```python
from build123d import *

# Parameters (mm, degrees)
F1_DEPTH = 12.7
F2_SIZE  = 12.7
F4_R     = 1.9812
F4_R_2   = 2.067369
F4_R_3   = 1.772036
F4_R_4   = 2.051504
F5_DEPTH = 12.701
F6_R     = 2.54
F7_DEPTH = 12.701


with BuildPart() as f1:
    # F0 (on Front) → F1 (new body)
    with BuildSketch(Plane.XZ):
        with BuildLine():
            Line((0, 25.4), (0, 0))
            Line((0, 0), (762, 0))
            Line((762, 0), (762, 562.7624))
            Line((762, 562.7624), (0, 562.7624))
            Line((0, 562.7624), (0, 537.3624))
            ThreePointArc((0, 537.3624), (-37.197439, 447.559839), (-127, 410.3624))
            Line((-127, 410.3624), (-711.2, 410.3624))
            Line((-711.2, 410.3624), (-711.2, 152.4))
            Line((-711.2, 152.4), (-127, 152.4))
            ThreePointArc((-127, 152.4), (-37.197439, 115.202561), (0, 25.4))
        make_face()
    extrude(amount=F1_DEPTH)

    # F2
    f2_edges = [f1.edges().sort_by_distance(p)[0] for p in [
        (-711.2, -6.35, 410.3624),
        (-711.2, -6.35, 152.4),
        (0, -6.35, 0),
        (0, -6.35, 562.7624),
        (762, -6.35, 562.7624),
        (762, -6.35, 0),
    ]]
    chamfer(f2_edges, length=F2_SIZE)

    # F4 (on face) → F5 (cut, through all)
    with BuildSketch(Plane.XZ.offset(12.7)):
        with Locations((713.74, 7.62)):
            Circle(F4_R)
        with Locations((739.14, 7.62)):
            Circle(F4_R_2)
        with Locations((739.14, 50.8)):
            Circle(F4_R_3)
        with Locations((713.74, 50.8)):
            Circle(F4_R_4)
        with Locations((713.74, 555.1424)):
            Circle(F4_R)
        with Locations((739.14, 555.1424)):
            Circle(F4_R)
        with Locations((739.14, 511.9624)):
            Circle(F4_R)
        with Locations((713.74, 511.9624)):
            Circle(F4_R)
        with Locations((22.86, 555.1424)):
            Circle(F4_R)
        with Locations((48.26, 555.1424)):
            Circle(F4_R)
        with Locations((48.26, 511.9624)):
            Circle(F4_R)
        with Locations((22.86, 511.9624)):
            Circle(F4_R)
        with Locations((22.86, 7.62)):
            Circle(F4_R)
        with Locations((48.26, 7.62)):
            Circle(F4_R)
        with Locations((48.26, 48.8188)):
            Circle(F4_R)
        with Locations((22.86, 48.8188)):
            Circle(F4_R)
    extrude(amount=-F5_DEPTH, mode=Mode.SUBTRACT)

    # F6 (on face) → F7 (cut, through all)
    with BuildSketch(Plane.XZ.offset(12.7)):
        with Locations((-703.58, 387.4008)):
            Circle(F6_R)
        with Locations((-685.8, 387.4008)):
            Circle(F6_R)
        with Locations((20.32, 387.4008)):
            Circle(F6_R)
        with Locations((38.1, 387.4008)):
            Circle(F6_R)
        with Locations((-703.58, 179.1208)):
            Circle(F6_R)
        with Locations((-683.26, 179.1208)):
            Circle(F6_R)
        with Locations((20.32, 179.1208)):
            Circle(F6_R)
        with Locations((38.1, 179.1208)):
            Circle(F6_R)
    extrude(amount=-F7_DEPTH, mode=Mode.SUBTRACT)


solid = f1.part
```
Geometry check sheet. Reference: the model listing, model coordinates, mm. Give positions to 0.01 mm unless a question says otherwise; leave off trailing zeros. Order: outer loops, then holes, each group sorted by start corner. A loop starts at its lowest first (then second) coordinate and runs counter-clockwise, first axis right, second up.
1. Section check C-C, the plane z = 445.5. Enter the section's corners in (x, y).
2. Thickness scan on L1, parallel to Z at x = 713.74, y = -8; L2, parallel to Z at x = 48.26, y = -8.5; L3, parallel to Z at x = 20.32, y = -10. Record the ranges inside material, lowest first.
3. Gauge pin test, flat ends, axial feed: pin 1 Ø3.5 at (x, z) = (739.14, 7.62) entering from -Y; pin 2 Ø6.5 at (y, z) = (-6, 541.5) entering from -X; pin 3 Ø4.5 at (x, z) = (713.74, 50.8) entering from +Y; pin 4 Ø2 at (y, z) = (-10.5, 405) entering from -X. Record the tip position at first contact, or that the pin passes through.
4. Section check A-A, the plane x = -250. Enter the section's corners in (y, z), and give its area (3 significant figures).
5. Section check B-B, the plane y = -3. Give the number of separate pieces and of enclosed holes in the cut face, and give its area (3 significant figures).
Values follow:
1. outline: (-39.31, -12.7) - (762, -12.7) - (762, 0) - (-39.31, 0) - close
2. L1: z = 0 to 5.64, 9.6 to 48.75, 52.85 to 509.98, 513.94 to 553.16, 557.12 to 562.76
2. L2: z = 0 to 5.64, 9.6 to 46.84, 50.8 to 509.98, 513.94 to 553.16, 557.12 to 562.76
2. L3: z = 0 to 176.58, 181.66 to 384.86, 389.94 to 562.76
3. pin 1: passes through
3. pin 2: stops at x = 0
3. pin 3: stops at y = 0
3. pin 4: stops at x = -704.86
4. outline: (-12.7, 152.4) - (0, 152.4) - (0, 410.36) - (-12.7, 410.36) - close
4. area: 3,280 mm2
5. separate pieces: 1
5. enclosed holes: 24
5. area: 618,000 mm2
